from build123d import *

# Parameters (mm, degrees)
BOSS_EXTRUDE1_DEPTH = 1.016
SKETCH2_OUTSIDE_W   = 58.782
SKETCH2_OUTSIDE_H   = 30.295
CUT_EXTRUDE1_DEPTH  = 36.715560747
FILLET1_R           = 1.5875


with BuildPart() as part:
    # Sketch1 → Boss-Extrude1 (new body)
    with BuildSketch(Plane.XY):
        with BuildLine():
            Line((-23.371860585, 13.49375), (-15.122968614, 8.73125))
            ThreePointArc((-15.122968614, 8.73125), (0, 17.4625), (15.122968614, 8.73125))
            Line((15.122968614, 8.73125), (23.371860585, 13.49375))
            ThreePointArc((23.371860585, 13.49375), (0, 26.9875), (-23.371860585, 13.49375))
        make_face()
    extrude(amount=BOSS_EXTRUDE1_DEPTH)

    # Sketch2 outside → Cut-Extrude1 (cut, through all)
    with BuildSketch(Plane.XY.offset(1.016)):
        with Locations((0, 17.8595)):
            Rectangle(SKETCH2_OUTSIDE_W, SKETCH2_OUTSIDE_H)
        with BuildLine():
            Line((-16.11283565, 9.30275), (-15.122968614, 8.73125))
            ThreePointArc((-15.122968614, 8.73125), (0, 17.4625), (15.122968614, 8.73125))
            Line((15.122968614, 8.73125), (16.11283565, 9.30275))
            ThreePointArc((16.11283565, 9.30275), (0, 26.9875), (-16.11283565, 9.30275))
        make_face(mode=Mode.SUBTRACT)
    extrude(amount=-CUT_EXTRUDE1_DEPTH, mode=Mode.SUBTRACT)

    # Fillet1
    fillet1_edges = [part.edges().sort_by_distance(p)[0] for p in [
        (16.11283565, 9.30275, 0.508),
        (-16.11283565, 9.30275, 0.508),
    ]]
    fillet(fillet1_edges, radius=FILLET1_R)


solid = part.part
Input: part model. Units: mm. Frame: model coordinates. Give positions to 0.01 mm unless a question says otherwise; leave off trailing zeros. Order: outer loops, then holes, each group sorted by start corner. A loop starts at its lowest first (then second) coordinate and runs counter-clockwise, first axis right, second up. Notation, with made-up numbers: (21.25, 11) -> (39.25, 11) arc R14 cw to (39.25, 33) -> close; hole circle Ø7 at (5.5, -10). An arc over 180 degrees is marked (long way). Use one line per item in the form item = value.
1) Section C-C, the plane x = 0. Return loops of the section in (y, z).
Response values:
outline = (17.46, 0) -> (26.99, 0) -> (26.99, 1.02) -> (17.46, 1.02) -> close
2) Section B-B, the plane x = -14. Return loops of the section in (y, z), and give its area (3 significant figures).
Response values:
outline = (10.44, 0) -> (18.92, 0) -> (18.92, 1.02) -> (10.44, 1.02) -> close
area = 8.62 mm^2
3) Mould query, pull axis X, two halves, no side actions, for faces 1 (the flat face through (0, 20, 0)), 2 (the cylindrical face through (-0.26, 17.46, 0.5)), 3 (the cylindrical face through (15.95, 9.44, 0.5)). Classes: pulls with the +X half, pulls with the -X half, needs draft (parallel to the pull), parting line crosses it, or undercut.
Response values:
face_1 = needs draft
face_2 = undercut
face_3 = pulls with the +X half
4) Line query: probe 1 along X at (y, z) = (16, 0.5); probe 2 along X at (y, z) = (23.5, 0.25); probe 3 along X at (y, z) = (12.75, 0.45). Output: solid intervals per line, ascending.
Response values:
probe_1 = -15.33 to -7, 7 to 15.33
probe_2 = -10.04 to 10.04
probe_3 = -16.07 to -11.93, 11.93 to 16.07
